Design review of the part built by this model. Coordinates are the model's own, in mm. Face numbers are marked on the shaded views. Give positions to 0.01 mm unless a question says otherwise; leave off trailing zeros. Loops run counter-clockwise (first coordinate to the right, second up) from the corner with the lowest first, then second, coordinate; pieces in that order, holes last. Notation, with made-up numbers: M 75,6.5 L 128,6.5 A12 ccw 128,16.5 Z; hole C -36,65.5 d3. An arc over 180 degrees is marked long. Use a Markdown table: item, result. Add a question column.
(1) Add section C-C, the plane y = -8.25. Give the boundary of the cut face in (x, z).
(2) For probe 1 along Y at (x, z) = (6, -7.25); probe 2 along Y at (x, z) = (13, 0.25); probe 3 along Z at (x, y) = (3.5, -7), list the stretches that pass through material, from the lowest coordinate up.
(3) Insertion check: pin 1 Ø3 at (x, z) = (2.5, 0) entering from -Y; pin 2 Ø6 at (x, z) = (10, -2.5) entering from +Y; pin 3 Ø3.5 at (x, y) = (7, -0.5) entering from +Z. Each pin has a flat end and moves straight along its axis. Give the tip position at first contact, or say it passes through.
(4) Add section A-A, the plane z = -6.25. Give the boundary of the cut face in (x, y).
(5) Add section B-B, the plane z = 0.25. Give the boundary of the cut face in (x, y).
(6) Draft analysis for pull direction Y (two halves, no side actions). For the marked faces 1 and 2, state which applies: pulls with the +Y half, pulls with the -Y half, needs draft (parallel to the pull), parting line crosses it, or undercut.
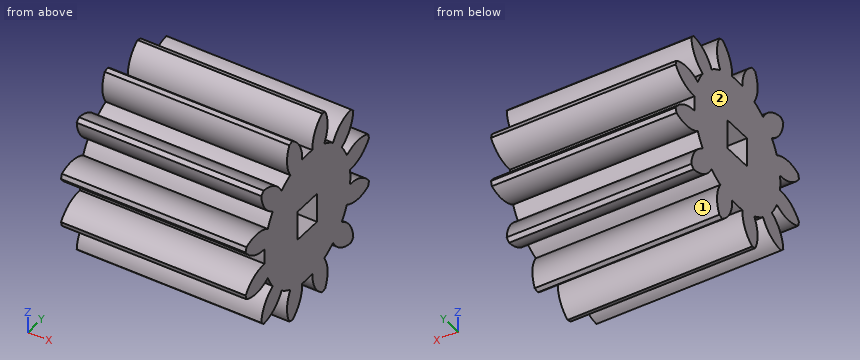
```python
from build123d import *

# Parameters (mm, degrees)
BASPROSKE_W        = 20
BASPROSKE_H        = 10.5
TOOTHCUT_DEPTH     = 25.909837414
TEETHCUTS_COUNT    = 12
TEETHCUTS_ANGLE    = 330
BORSKE_R           = 0.5
BORE_DEPTH         = 50.0000508
SKETCH1_W          = 3.2
SKETCH1_H          = 3.2
CUT_EXTRUDE1_DEPTH = 30


with BuildPart() as part:
    # BasProSke → Base-Revolve (revolve)
    with BuildSketch(Plane(origin=(0, 0, 0), x_dir=(1, 0, 0), z_dir=(0, 1, 0)), mode=Mode.PRIVATE) as base_revolve_sk:
        with Locations((10, 5.25)):
            Rectangle(BASPROSKE_W, BASPROSKE_H)
    revolve(base_revolve_sk.sketch.rotate(Axis((-10, 0, 0), (1, 0, 0)), 180), axis=Axis((-10, 0, 0), (1, 0, 0)))

    # TooCutSke → ToothCut (cut, through all)
    with BuildSketch(Plane(origin=(0, 0, 0), x_dir=(0, 0, -1), z_dir=(1, 0, 0))):
        with BuildLine():
            ThreePointArc((0.837751456, 7.074570552), (0, 7.124), (-0.837751456, 7.074570552))
            ThreePointArc((-0.837751456, 7.074570552), (-1.245380016, 8.868946541), (-2.486473743, 10.227487154))
            ThreePointArc((-2.486473743, 10.227487154), (0, 10.5254), (2.486473743, 10.227487154))
            ThreePointArc((2.486473743, 10.227487154), (1.245380016, 8.868946541), (0.837751456, 7.074570552))
        make_face()
    toothcut = extrude(amount=TOOTHCUT_DEPTH, mode=Mode.SUBTRACT)

    # TeethCuts: ToothCut ×12 about axis
    teethcuts_axis = Axis((-10, 0, 0), (1, 0, 0))
    for i in range(1, TEETHCUTS_COUNT):
        add(toothcut.rotate(teethcuts_axis, i * TEETHCUTS_ANGLE / (TEETHCUTS_COUNT - 1)), mode=Mode.SUBTRACT)

    # BorSke → Bore (cut, symmetric)
    with BuildSketch(Plane(origin=(0, 0, 0), x_dir=(0, 0, -1), z_dir=(1, 0, 0))):
        with Locations(Location((0, 0, 0), (0, 0, 180))):
            Circle(BORSKE_R)
    extrude(amount=BORE_DEPTH, both=True, mode=Mode.SUBTRACT)

    # Sketch1 → Cut-Extrude1 (cut)
    with BuildSketch(Plane(origin=(20, 0, 0), x_dir=(0, 0, -1), z_dir=(1, 0, 0))):
        Rectangle(SKETCH1_W, SKETCH1_H)
    extrude(amount=-CUT_EXTRUDE1_DEPTH, mode=Mode.SUBTRACT)


solid = part.part
```
Established:
| question | item | result |
|---|---|---|
| 1 | outline | M 0,-3.35 L 20,-3.35 L 20,-0.99 L 0,-0.99 Z; M 0,0.99 L 20,0.99 L 20,3.35 L 0,3.35 Z |
| 2 | probe 1 | -7.6 to -5.86, -3.15 to -0.84, 0.84 to 3.15, 5.86 to 7.6 |
| 2 | probe 2 | -7.12 to -1.6, 1.6 to 7.12 |
| 2 | probe 3 | -7.59 to -5.42, -3.05 to 3.05, 5.42 to 7.59 |
| 3 | pin 1 | y = -9.28 |
| 3 | pin 2 | y = 10.21 |
| 3 | pin 3 | z = 10.06 |
| 4 | outline | M 0,-7.42 L 20,-7.42 L 20,-4.62 L 0,-4.62 Z; M 0,-3.42 L 20,-3.42 L 20,3.42 L 0,3.42 Z; M 0,4.62 L 20,4.62 L 20,7.42 L 0,7.42 Z |
| 5 | outline | M 0,-7.12 L 20,-7.12 L 20,-1.6 L 0,-1.6 Z; M 0,1.6 L 20,1.6 L 20,7.12 L 0,7.12 Z |
| 6 | face 1 | undercut |
| 6 | face 2 | needs draft |
